For this review, take the finished solid that the model builds, in its own axes (mm). A direction names the side the tool comes from. Coordinates: 2 decimals unless noted, no trailing zeros. Write each loop counter-clockwise with the first axis right and the second up, starting at its lowest first coordinate (ties: lowest second). Pieces come first, ordered by that corner, then holes. Notation, with made-up numbers: M 28.25,65 L 53.25,65 A9 ccw 53.25,70 Z; hole C 35.25,30 d5. An arc over 180 degrees is marked long. One line per question, with ' | ' between items.
from build123d import *

# Parameters (mm, degrees)
BOSS_EXTRUDE1_DEPTH = 3.175
FILLET1_R           = 7
FILLET2_R           = 5
SKETCH2_R           = 3.175
CUT_EXTRUDE1_DEPTH  = 52.721181589
LPATTERN1_COUNT     = 3
LPATTERN1_PITCH     = 12.5


with BuildPart() as part:
    # Sketch1 → Boss-Extrude1 (new body)
    with BuildSketch(Plane.XY):
        with BuildLine():
            Line((-11.618950039, 11), (-36, 11))
            Line((-36, 11), (-36, -26))
            ThreePointArc((-36, -26), (-25, -37), (-14, -26))
            Line((-14, -26), (-14, -11))
            Line((-14, -11), (-11.618950039, -11))
            ThreePointArc((-11.618950039, -11), (16, 0), (-11.618950039, 11))
        make_face()
    extrude(amount=BOSS_EXTRUDE1_DEPTH)

    # Fillet1
    fillet1_edges = [part.edges().sort_by_distance(p)[0] for p in [
        (-36, 11, 1.5875),
    ]]
    fillet(fillet1_edges, radius=FILLET1_R)

    # Fillet2
    # the kernel refuses this fillet: 5 mm, written as the material it adds along each edge
    with BuildSketch(Plane(origin=(-14, -11, 0), x_dir=(1, 0, 0), z_dir=(0, 0, 1))) as fillet2_piece_1:
        with BuildLine():
            CenterArc((5, -4.259237102), FILLET2_R, 121.586822832, 58.413177168)
            Line((0, -4.259237102), (-0.1, -4.259237102))
            Line((-0.1, -4.259237102), (-0.1, 0))
            Line((-0.1, 0), (0, 0.1))
            ThreePointArc((0, 0.1), (1.190524981, 0.1), (2.328670961, 0.085184742))
            Line((2.328670961, 0.085184742), (2.381049961, 0))
        make_face()
    extrude(amount=3.175)

    # Sketch2 → Cut-Extrude1 (cut, through all)
    with BuildSketch(Plane.XY.offset(3.175)):
        Circle(SKETCH2_R)
    cut_extrude1 = extrude(amount=-CUT_EXTRUDE1_DEPTH, mode=Mode.SUBTRACT)

    # LPattern1: Cut-Extrude1 ×3
    with Locations(*[(-i * LPATTERN1_PITCH, 0, 0) for i in range(1, LPATTERN1_COUNT)]):
        add(cut_extrude1, mode=Mode.SUBTRACT)


solid = part.part
1) We need section B-B on x = -25. State the section outline as (y, z) points (3 decimals).
Responses:
outline: M -37,0 L -3.175,0 L -3.175,3.175 L -37,3.175 Z; M 3.175,0 L 11,0 L 11,3.175 L 3.175,3.175 Z
2) To check wall thickness, follow line 1 along Y through (x, z) = (-25, 0.9) (3 decimals); line 2 along X through (y, z) = (-2.5, 0.3); line 3 along Y through (x, z) = (0, 2.2) (3 decimals). State the ranges of each line that lie inside material, in increasing order. Write a range as [from, to].
Responses:
line 1: [-37, -3.175], [3.175, 11] | line 2: [-36, -26.96], [-23.04, -14.46], [-10.54, -1.96], [1.96, 15.8] | line 3: [-16, -3.175], [3.175, 16]
3) We need section D-D on x = 0. State the section outline as (y, z) points (3 decimals), then the cut area to 3 significant figures.
Responses:
outline: M -16,0 L -3.175,0 L -3.175,3.175 L -16,3.175 Z; M 3.175,0 L 16,0 L 16,3.175 L 3.175,3.175 Z | area: 81.4 mm^2
4) Machinability: for faces 1 (the cylindrical face through (-0.69, -3.1, 1.61)), 2 (the flat face through (-20, 11, 2)), which of the approach directions +Z, -Z, +X, -X, +Y, -Y give a long, thin tool a straight path to every point of the face, cutting with its end or side? Answer none if there is none.
Responses:
face 1: +Z, -Z | face 2: +Z, -Z, -X, +Y
5) We need section C-C on z = 1.05. State the section outline as (x, y) points (3 decimals).
Responses:
outline: M -36,-26 A11 ccw -14,-26 L -14,-15.259 A5 cw -11.619,-11 A16 ccw long -11.619,11 L -29,11 A7 ccw -36,4 Z; hole C -25,0 d6.35; hole C -12.5,0 d6.35; hole C 0,0 d6.35
6) We need section A-A on y = 0. State the section outline as (x, z) points (3 decimals), then the cut area to 3 significant figures.
Responses:
outline: M -36,0 L -28.175,0 L -28.175,3.175 L -36,3.175 Z; M -21.825,0 L -15.675,0 L -15.675,3.175 L -21.825,3.175 Z; M -9.325,0 L -3.175,0 L -3.175,3.175 L -9.325,3.175 Z; M 3.175,0 L 16,0 L 16,3.175 L 3.175,3.175 Z | area: 105 mm^2
7) Insertion check: pin 1 Ø1 at (x, z) = (-22, 2) entering from +Y; pin 2 Ø1.5 at (x, z) = (-16, 2) entering from -Y. Each pin has a flat end and moves straight along its axis. Give the tip position at first contact, or say it passes through.
Responses:
pin 1: y = 11 | pin 2: y = -33.28
8) The part is to be moulded in two halves that separate along X. For faces 3 (the cylindrical face through (-28.17, 0.14, 1.61)), 4 (the cylindrical face through (-13.35, -12.79, 1.57)), 5 (the cylindrical face through (-33.9, 9, 1.6)), 6 (the flat face through (-15, -4, 3.175)), say which applies: +X half, -X half, draft (parallel to the pull), parting line (faces both ways), or undercut.
Responses:
face 3: undercut | face 4: undercut | face 5: -X half | face 6: draft
